The model under review builds one solid part; all positions refer to its coordinate system, in mm. A direction names the side the tool comes from. Round coordinates to 2 decimals unless told otherwise and drop trailing zeros. Write each loop counter-clockwise with the first axis right and the second up, starting at its lowest first coordinate (ties: lowest second). Pieces come first, ordered by that corner, then holes.
Item 1: Machinability: for faces 1 (the face through (96, 59, 20)), 2 (the face through (1, 33, 82)), 3 (the face through (59, 1, 83)), 4 (the face through (119, 33, 83)), which of the approach directions +Z, -Z, +X, -X, +Y, -Y give a long, thin tool a straight path to every point of the face, cutting with its end or side? Answer none if there is none.
Item 2: Add section D-D (z = 11). Give the boundary of the cut face in (x, y).
Item 3: Add section C-C (x = 81.5). Give the boundary of the cut face in (y, z).
Item 4: Clearance check with flat-ended pins moving along their axes: pin 1 Ø5 at (x, y) = (61.5, 57.5) entering from +Z; pin 2 Ø1.5 at (x, z) = (54.5, 82) entering from -Y; pin 3 Ø1.5 at (y, z) = (17, 83) entering from +X. State where each tip first meets the part, or that it passes through.
Item 5: To check wall thickness, follow L1, parallel to X at y = 59, z = 7.5; L2, parallel to X at y = 60, z = 8; L3, parallel to Y at x = 12, z = 43. State the ranges of each line that lie inside material, in increasing order.
Item 6: Add section B-B (y = 44.5). Give the boundary of the cut face in (x, z).
Item 7: Add section A-A (z = 63). Give the boundary of the cut face in (x, y).
Item 8: Draft analysis for pull direction Y (two halves, no side actions). For faces 5 (the face through (60, 63, 85)), 6 (the face through (59, 0, 39)), 7 (the face through (92, 52.5, 18)), 8 (the face through (59, 33, 3)), state which applies: +Y half, -Y half, draft (parallel to the pull), parting line (faces both ways), or undercut.
```python
from build123d import *

# Parameters (mm, degrees)
SKETCH2_W           = 120
SKETCH2_H           = 65
BOSS_EXTRUDE1_DEPTH = 85
SKETCH3_W           = 115
SKETCH3_H           = 60
CUT_EXTRUDE1_DEPTH  = 82
SKETCH4_W           = 5
SKETCH4_H           = 65
CUT_EXTRUDE2_DEPTH  = 1
SKETCH5_W           = 119
SKETCH5_H           = 5
CUT_EXTRUDE3_DEPTH  = 1
BOSS_EXTRUDE2_DEPTH = 85
SKETCH9_W           = 5
SKETCH9_H           = 64
CUT_EXTRUDE4_DEPTH  = 1
SKETCH10_W          = 118
SKETCH10_H          = 5
CUT_EXTRUDE5_DEPTH  = 1
SKETCH11_W          = 42
SKETCH11_H          = 14
CUT_EXTRUDE6_DEPTH  = 10
SKETCH12_W          = 42.071261004
SKETCH12_H          = 10
BOSS_EXTRUDE3_DEPTH = 4
SKETCH13_W          = 2
SKETCH13_H          = 10
BOSS_EXTRUDE4_DEPTH = 17
SKETCH14_W          = 44.402934601
SKETCH14_H          = 10
BOSS_EXTRUDE5_DEPTH = 2
SKETCH15_W          = 44.064994884
SKETCH15_H          = 8
BOSS_EXTRUDE6_DEPTH = 2
SKETCH16_W          = 2
SKETCH16_H          = 2
BOSS_EXTRUDE7_DEPTH = 12
SKETCH17_W          = 17
SKETCH17_H          = 4
CUT_EXTRUDE7_DEPTH  = 5


with BuildPart() as part:
    # Sketch2 → Boss-Extrude1 (new body)
    with BuildSketch(Plane.XY):
        with Locations((60, 32.5)):
            Rectangle(SKETCH2_W, SKETCH2_H)
    extrude(amount=BOSS_EXTRUDE1_DEPTH)

    # Sketch3 → Cut-Extrude1 (cut)
    with BuildSketch(Plane.XY.offset(85)):
        with Locations((60, 32.5)):
            Rectangle(SKETCH3_W, SKETCH3_H)
    extrude(amount=-CUT_EXTRUDE1_DEPTH, mode=Mode.SUBTRACT)

    # Sketch4 → Cut-Extrude2 (cut)
    with BuildSketch(Plane.ZY):
        with Locations((82.5, 32.5)):
            Rectangle(SKETCH4_W, SKETCH4_H)
    extrude(amount=-CUT_EXTRUDE2_DEPTH, mode=Mode.SUBTRACT)

    # Sketch5 → Cut-Extrude3 (cut)
    with BuildSketch(Plane(origin=(0, 65, 0), x_dir=(1, 0, 0), z_dir=(0, 1, 0))):
        with Locations((60.5, -82.5)):
            Rectangle(SKETCH5_W, SKETCH5_H)
    extrude(amount=-CUT_EXTRUDE3_DEPTH, mode=Mode.SUBTRACT)

    # Sketch7 → Boss-Extrude2 (add)
    with BuildSketch(Plane.XY.offset(85)):
        Polygon((2.5, 62.5), (2.5, 59.5), (5.5, 62.5), align=None)
        Polygon((117.5, 62.5), (114.5, 62.5), (117.5, 59.5), align=None)
        Polygon((117.5, 5.5), (117.5, 2.5), (114.5, 2.5), align=None)
        Polygon((2.5, 2.5), (2.5, 5.5), (5.5, 2.5), align=None)
    extrude(amount=-BOSS_EXTRUDE2_DEPTH)

    # Sketch9 → Cut-Extrude4 (cut)
    with BuildSketch(Plane(origin=(120, 0, 0), x_dir=(0, 0, -1), z_dir=(1, 0, 0))):
        with Locations((-82.5, 32)):
            Rectangle(SKETCH9_W, SKETCH9_H)
    extrude(amount=-CUT_EXTRUDE4_DEPTH, mode=Mode.SUBTRACT)

    # Sketch10 → Cut-Extrude5 (cut)
    with BuildSketch(Plane.XZ):
        with Locations((60, 82.5)):
            Rectangle(SKETCH10_W, SKETCH10_H)
    extrude(amount=-CUT_EXTRUDE5_DEPTH, mode=Mode.SUBTRACT)

    # Sketch11 → Cut-Extrude6 (cut)
    with BuildSketch(Plane(origin=(0, 65, 0), x_dir=(1, 0, 0), z_dir=(0, 1, 0))):
        with Locations((96.5, -13)):
            Rectangle(SKETCH11_W, SKETCH11_H)
    extrude(amount=-CUT_EXTRUDE6_DEPTH, mode=Mode.SUBTRACT)

    # Sketch12 → Boss-Extrude3 (add)
    with BuildSketch(Plane.XY.offset(6)):
        with Locations((96.535630502, 57.5)):
            Rectangle(SKETCH12_W, SKETCH12_H)
    extrude(amount=-BOSS_EXTRUDE3_DEPTH)

    # Sketch13 → Boss-Extrude4 (add)
    with BuildSketch(Plane.XY.offset(3)):
        with Locations((74.5, 57.5)):
            Rectangle(SKETCH13_W, SKETCH13_H)
    extrude(amount=BOSS_EXTRUDE4_DEPTH)

    # Sketch14 → Boss-Extrude5 (add)
    with BuildSketch(Plane.XY.offset(20)):
        with Locations((95.701467301, 57.5)):
            Rectangle(SKETCH14_W, SKETCH14_H)
    extrude(amount=BOSS_EXTRUDE5_DEPTH)

    # Sketch15 → Boss-Extrude6 (add)
    with BuildSketch(Plane.XZ.offset(-52.5)):
        with Locations((95.532497442, 18)):
            Rectangle(SKETCH15_W, SKETCH15_H)
    extrude(amount=BOSS_EXTRUDE6_DEPTH)

    # Sketch16 → Boss-Extrude7 (add)
    with BuildSketch(Plane.XY.offset(3)):
        with Locations((74.5, 51.5)):
            Rectangle(SKETCH16_W, SKETCH16_H)
    extrude(amount=BOSS_EXTRUDE7_DEPTH)

    # Sketch17 → Cut-Extrude7 (cut)
    with BuildSketch(Plane(origin=(0, 52.5, 0), x_dir=(1, 0, 0), z_dir=(0, 1, 0))):
        with Locations((106.612593264, -16)):
            Rectangle(SKETCH17_W, SKETCH17_H)
    extrude(amount=-CUT_EXTRUDE7_DEPTH, mode=Mode.SUBTRACT)


solid = part.part
```
Numbers:
1. face 1: +Y
1. face 2: +Z, -X, +Y, -Y
1. face 3: +Z, +X, -X, -Y
1. face 4: +Z, +X, +Y, -Y
2. outline: (0, 0) - (120, 0) - (120, 65) - (117.5, 65) - (117.5, 5.5) - (114.5, 2.5) - (5.5, 2.5) - (2.5, 5.5) - (2.5, 59.5) - (5.5, 62.5) - (73.5, 62.5) - (73.5, 50.5) - (75.5, 50.5) - (75.5, 65) - (0, 65) - close
3. outline: (0, 0) - (65, 0) - (65, 6) - (52.5, 6) - (52.5, 3) - (2.5, 3) - (2.5, 85) - (1, 85) - (1, 80) - (0, 80) - close; (50.5, 14) - (52.5, 14) - (52.5, 20) - (65, 20) - (65, 80) - (64, 80) - (64, 85) - (62.5, 85) - (62.5, 22) - (50.5, 22) - close
4. pin 1: stops at z = 3
4. pin 2: stops at y = 1
4. pin 3: stops at x = 119
5. L1: x = 0 to 2.5, 73.5 to 75.5, 117.5 to 120
5. L2: x = 0 to 3, 73.5 to 75.5, 117.5 to 120
5. L3: y = 0 to 2.5, 62.5 to 65
6. outline: (0, 0) - (120, 0) - (120, 80) - (119, 80) - (119, 85) - (117.5, 85) - (117.5, 3) - (2.5, 3) - (2.5, 85) - (1, 85) - (1, 80) - (0, 80) - close
7. outline: (0, 0) - (120, 0) - (120, 65) - (0, 65) - close; hole (2.5, 5.5) - (5.5, 2.5) - (114.5, 2.5) - (117.5, 5.5) - (117.5, 59.5) - (114.5, 62.5) - (5.5, 62.5) - (2.5, 59.5) - close
8. face 5: draft
8. face 6: -Y half
8. face 7: +Y half
8. face 8: undercut
